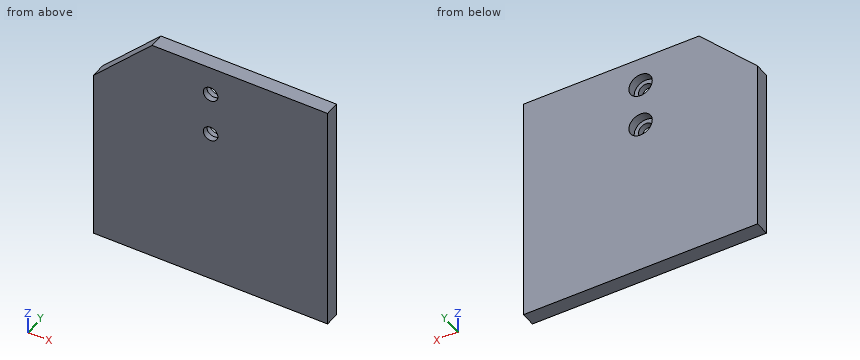
```python
from build123d import *

# Parameters (mm, degrees)
BOSS_EXTRUDE1_DEPTH = 5
SKETCH2_R           = 2.5
CUT_EXTRUDE1_DEPTH  = 15
SKETCH3_R           = 4
CUT_EXTRUDE2_DEPTH  = 3


with BuildPart() as part:
    # Sketch1 → Boss-Extrude1 (new body)
    with BuildSketch(Plane(origin=(0, 0, 0), x_dir=(1, 0, 0), z_dir=(0, 1, 0))):
        Polygon((40, -40), (-20, -40), (-40, -20), (-40, 40), (40, 40), align=None)
    extrude(amount=BOSS_EXTRUDE1_DEPTH)

    # Sketch2 → Cut-Extrude1 (cut)
    with BuildSketch(Plane(origin=(0, 5, 0), x_dir=(1, 0, 0), z_dir=(0, 1, 0))):
        with Locations(Location((0, -15, 0), (0, 0, 270))):
            Circle(SKETCH2_R)
        with Locations(Location((0, -30, 0), (0, 0, 270))):
            Circle(SKETCH2_R)
    extrude(amount=-CUT_EXTRUDE1_DEPTH, mode=Mode.SUBTRACT)

    # Sketch3 → Cut-Extrude2 (cut)
    with BuildSketch(Plane(origin=(0, 5, 0), x_dir=(1, 0, 0), z_dir=(0, 1, 0))):
        with Locations(Location((0, -15, 0), (0, 0, 270))):
            Circle(SKETCH3_R)
        with Locations(Location((0, -30, 0), (0, 0, 270))):
            Circle(SKETCH3_R)
    extrude(amount=-CUT_EXTRUDE2_DEPTH, mode=Mode.SUBTRACT)


solid = part.part
```
Can you work these out from the model? Positions are in its coordinate system, mm. Give positions to 0.01 mm unless a question says otherwise; leave off trailing zeros. Order: outer loops, then holes, each group sorted by start corner. A loop starts at its lowest first (then second) coordinate and runs counter-clockwise, first axis right, second up. Notation, with made-up numbers: M -34,66.25 L 8,66.25 A18 cw 8,74.25 Z; hole C 77,-40 d4. An arc over 180 degrees is marked long. Write item = value, one per line. Start each with the question number.
Q1. Will these pins go through, and if not, where does the flat tip stop? pin 1 Ø6.5 at (x, z) = (0, 30) entering from +Y; pin 2 Ø3 at (x, z) = (0, 15) entering from +Y.
Q2. Suppose I cut it at C-C (z = 15). Write out the boundary of the cut face in (x, y).
Q3. Suppose I cut it at D-D (x = -24). Write out the boundary of the cut face in (y, z).
Q4. I need wall thicknesses on probe 1 along X at (y, z) = (0.95, 15); probe 2 along X at (y, z) = (3.6, 15); probe 3 along Z at (x, y) = (-3, 3.3). Which ranges of each line are inside material? Lowest first, please. Write a range as [from, to].
Q5. Suppose I cut it at B-B (x = 0). Write out the boundary of the cut face in (y, z), plus the area to 3 significant figures.
Q6. Suppose I cut it at A-A (z = 30). Write out the boundary of the cut face in (x, y), plus the area to 3 significant figures.
Check result:
q1.pin_1 = 2
q1.pin_2 = through
q2.outline = M -40,0 L -2.5,0 L -2.5,2 L -4,2 L -4,5 L -40,5 Z; M 2.5,0 L 40,0 L 40,5 L 4,5 L 4,2 L 2.5,2 Z
q3.outline = M 0,-40 L 5,-40 L 5,36 L 0,36 Z
q4.probe_1 = [-40, -2.5], [2.5, 40]
q4.probe_2 = [-40, -4], [4, 40]
q4.probe_3 = [-40, 12.35], [17.65, 27.35], [32.65, 40]
q5.outline = M 0,-40 L 5,-40 L 5,11 L 2,11 L 2,12.5 L 0,12.5 Z; M 0,17.5 L 2,17.5 L 2,19 L 5,19 L 5,26 L 2,26 L 2,27.5 L 0,27.5 Z; M 0,32.5 L 2,32.5 L 2,34 L 5,34 L 5,40 L 0,40 Z
q5.area = 332 mm2
q6.outline = M -30,0 L -2.5,0 L -2.5,2 L -4,2 L -4,5 L -30,5 Z; M 2.5,0 L 40,0 L 40,5 L 4,5 L 4,2 L 2.5,2 Z
q6.area = 316 mm2
